Geometry: final body of the model. Coordinates: model frame, mm. Give positions to 0.01 mm unless a question says otherwise; leave off trailing zeros. Order: outer loops, then holes, each group sorted by start corner. A loop starts at its lowest first (then second) coordinate and runs counter-clockwise, first axis right, second up. Notation, with made-up numbers: M -24,52.5 L -8,52.5 A4 cw -8,57.5 Z; hole C 42,59 d6. An arc over 180 degrees is marked long. Write item = value, one per line. Start each with the question number.
from build123d import *

# Parameters (mm, degrees)
EXTRUDE_1_DEPTH          = 5
SKETCH_2_R               = 1.7
CUT_EXTRUDE_1_DEPTH      = 5
PATTERN_CIRCULAR_1_COUNT = 3
SKETCH_3_R               = 11
SKETCH_3_R_2             = 1.7
CUT_EXTRUDE_2_DEPTH      = 10
SKETCH_4_R               = 1.7
CUT_EXTRUDE_3_DEPTH      = 10


with BuildPart() as part:
    # 草图1 → 凸台-拉伸1 (new body)
    with BuildSketch(Plane.XY):
        with BuildLine():
            Line((81.5, -28), (81.5, 28))
            ThreePointArc((81.5, 28), (80.621320344, 30.121320344), (78.5, 31))
            Line((78.5, 31), (58.889727457, 31))
            ThreePointArc((58.889727457, 31), (57.389727457, 31.401923789), (56.291651246, 32.5))
            ThreePointArc((56.291651246, 32.5), (-65, 0), (56.291651246, -32.5))
            ThreePointArc((56.291651246, -32.5), (57.389727457, -31.401923789), (58.889727457, -31))
            Line((58.889727457, -31), (78.5, -31))
            ThreePointArc((78.5, -31), (80.621320344, -30.121320344), (81.5, -28))
        make_face()
    extrude(amount=EXTRUDE_1_DEPTH)

    # 草图2 → 切除-拉伸1 (cut)
    with BuildSketch(Plane.XY.offset(5)):
        with Locations((58.34, 0)):
            Circle(SKETCH_2_R)
        with Locations((46.34, -12)):
            Circle(SKETCH_2_R)
        with Locations((34.34, 0)):
            Circle(SKETCH_2_R)
        with Locations((46.34, 12)):
            Circle(SKETCH_2_R)
    cut_extrude_1 = extrude(amount=-CUT_EXTRUDE_1_DEPTH, mode=Mode.SUBTRACT)

    # 阵列(圆周)1: 切除-拉伸1 ×3 about axis
    pattern_circular_1_axis = Axis((0, 0, 0), (0, 0, 1))
    for i in range(1, PATTERN_CIRCULAR_1_COUNT):
        add(cut_extrude_1.rotate(pattern_circular_1_axis, i * 360 / PATTERN_CIRCULAR_1_COUNT), mode=Mode.SUBTRACT)

    # 草图3 → 切除-拉伸2 (cut)
    with BuildSketch(Plane.XY.offset(5)):
        Circle(SKETCH_3_R)
        with Locations((15.5, -15.5)):
            Circle(SKETCH_3_R_2)
        with Locations((15.5, 15.5)):
            Circle(SKETCH_3_R_2)
        with Locations((-15.5, 15.5)):
            Circle(SKETCH_3_R_2)
        with Locations((-15.5, -15.5)):
            Circle(SKETCH_3_R_2)
        with Locations((72, 20)):
            Circle(SKETCH_3_R_2)
        with Locations((72, -20)):
            Circle(SKETCH_3_R_2)
    extrude(amount=-CUT_EXTRUDE_2_DEPTH, mode=Mode.SUBTRACT)

    # 草图4 → 切除-拉伸3 (cut)
    with BuildSketch(Plane.XY.offset(5)):
        with Locations((0, 28.5)):
            Circle(SKETCH_4_R)
        with Locations((24.681724008, 14.25)):
            Circle(SKETCH_4_R)
        with Locations((24.681724008, -14.25)):
            Circle(SKETCH_4_R)
        with Locations((0, -28.5)):
            Circle(SKETCH_4_R)
        with Locations((-24.681724008, -14.25)):
            Circle(SKETCH_4_R)
        with Locations((-24.681724008, 14.25)):
            Circle(SKETCH_4_R)
    extrude(amount=-CUT_EXTRUDE_3_DEPTH, mode=Mode.SUBTRACT)


solid = part.part
1) Cut plane A-A (x = 0). Return loops of the section in (y, z), plus the area to 3 significant figures.
2) Cut plane B-B (x = 34.34). Return loops of the section in (y, z).
3) Pin query (flat end, axial travel): pin 1 Ø2 at (x, y) = (-33.56, 34.13) entering from -Z; pin 2 Ø2 at (x, z) = (-10, 2) entering from +Y; pin 3 Ø1 at (x, z) = (-31, 2.5) entering from -Y; pin 4 Ø3 at (x, z) = (-5.5, 2) entering from -Y. Return the tip coordinate at first contact, or that it passes through.
4) Cut plane D-D (y = -20). Return loops of the section in (x, z).
5) Cut plane C-C (z = 2.05). Give the number of separate pieces and of enclosed holes in the cut face, plus the area to 3 significant figures.
6) Draft query along Y for faces 1 (the cylindrical face through (23, -14, 3)), 2 (the flat face through (69, -31, 2)), 3 (the flat face through (7, -14, 5)). Return one class per face: pulls with the +Y half, pulls with the -Y half, needs draft (parallel to the pull), parting line crosses it, or undercut.
7) Ray query, L1, parallel to Y at x = -29.17, z = 2.6; L2, parallel to Y at x = -30.5, z = 4; L3, parallel to Y at x = 67.5, z = 1.85. Return the intervals inside material, ascending.
Reply:
q1.outline = M -65,0 L -30.2,0 L -30.2,5 L -65,5 Z; M -26.8,0 L -11,0 L -11,5 L -26.8,5 Z; M 11,0 L 26.8,0 L 26.8,5 L 11,5 Z; M 30.2,0 L 65,0 L 65,5 L 30.2,5 Z
q1.area = 506 mm²
q2.outline = M -55.19,0 L -1.7,0 L -1.7,5 L -55.19,5 Z; M 1.7,0 L 55.19,0 L 55.19,5 L 1.7,5 Z
q3.pin_1 = through
q3.pin_2 = 64.37
q3.pin_3 = -57.4
q3.pin_4 = -64.88
q4.outline = M -61.85,0 L 70.3,0 L 70.3,5 L -61.85,5 Z; M 73.7,0 L 81.5,0 L 81.5,5 L 73.7,5 Z
q5.separate_pieces = 1
q5.enclosed_holes = 25
q5.area = 13,900 mm²
q6.face_1 = undercut
q6.face_2 = pulls with the -Y half
q6.face_3 = needs draft
q7.L1 = -58.09 to -52.22, -48.82 to 48.82, 52.22 to 58.09
q7.L2 = -57.4 to -51.58, -49.47 to 49.47, 51.58 to 57.4
q7.L3 = -31 to 31
